Can you work these out from the model? Positions are in its coordinate system, mm. A direction names the side the tool comes from. Give positions to 0.01 mm unless a question says otherwise; leave off trailing zeros. Loops run counter-clockwise (first coordinate to the right, second up) from the corner with the lowest first, then second, coordinate; pieces in that order, holes last. Notation, with made-up numbers: (13.25, 78) - (63.25, 78) arc R18 ccw to (63.25, 85) - close; hole circle Ø11 at (43, -21). An arc over 180 degrees is marked (long way). Write item = value, one per line.
from build123d import *

# Parameters (mm, degrees)
F0_R        = 2.61
F1_DEPTH    = 15
F2_R        = 7.5
F2_R_2      = 2.61
F3_DEPTH    = 5
F4_R        = 7.5
F4_R_2      = 2.61
F5_DEPTH    = 13.5
F6_R        = 7.5
F6_R_2      = 2.61
F7_DEPTH    = 21
F8_C1_SIZE2 = 0.5
F8_C1_SIZE  = 1
F8_C2_SIZE2 = 0.5
F8_C2_SIZE  = 1
F8_C3_SIZE2 = 1
F8_C3_SIZE  = 0.5
F8_C4_SIZE2 = 1
F8_C4_SIZE  = 0.5
F8_C5_SIZE2 = 1
F8_C5_SIZE  = 0.5
F8_C6_SIZE2 = 0.5
F8_C6_SIZE  = 1
F9_SIZE     = 1


with BuildPart() as f1:
    # F0 (on Top) → F1 (new body)
    with BuildSketch(Plane.XY):
        with BuildLine():
            Line((20.7144641229, 7.4945626465), (6.3477137036, 32.3785043124))
            ThreePointArc((6.3477137036, 32.3785043124), (0, 43.8730669589), (-6.3477137036, 32.3785043124))
            Line((-6.3477137036, 32.3785043124), (-20.7144641229, 7.4945626465))
            ThreePointArc((-20.7144641229, 7.4945626465), (-27.4951905284, -3.75), (-14.3667504193, -3.5))
            Line((-14.3667504193, -3.5), (14.3667504193, -3.5))
            ThreePointArc((14.3667504193, -3.5), (27.4951905284, -3.75), (20.7144641229, 7.4945626465))
        make_face()
        with Locations((-21, 0)):
            Circle(F0_R, mode=Mode.SUBTRACT)
        with Locations((21, 0)):
            Circle(F0_R, mode=Mode.SUBTRACT)
        Polygon((12.3397459622, 5), (-12.3397459622, 5), (0, 26.3730669589), align=None, mode=Mode.SUBTRACT)
        with Locations((0, 36.3730669589)):
            Circle(F0_R, mode=Mode.SUBTRACT)
    extrude(amount=F1_DEPTH)

    # F2 (on face) → F3 (join)
    with BuildSketch(Plane.XY.offset(15)):
        with Locations((0, 36.3730669589)):
            Circle(F2_R)
        with Locations((0, 36.3730669589)):
            Circle(F2_R_2, mode=Mode.SUBTRACT)
    extrude(amount=F3_DEPTH)

    # F4 (on face) → F5 (join)
    with BuildSketch(Plane.XY.offset(15)):
        with Locations((21, 0)):
            Circle(F4_R)
        with Locations((21, 0)):
            Circle(F4_R_2, mode=Mode.SUBTRACT)
    extrude(amount=F5_DEPTH)

    # F6 (on face) → F7 (join)
    with BuildSketch(Plane.XY.offset(15)):
        with Locations((-21, 0)):
            Circle(F6_R)
        with Locations((-21, 0)):
            Circle(F6_R_2, mode=Mode.SUBTRACT)
    extrude(amount=F7_DEPTH)

    # F8: chamfer of 0.5 x 1 on 6 edges, made by hand

    # F8_c1
    f8_c1_edges = [f1.edges().sort_by_distance(p)[0] for p in [
        (-23.61, 0, 36),
    ]]
    f8_c1_side = f1.faces().sort_by_distance((-23.62, 0, 36))[0]
    chamfer(f8_c1_edges, length=F8_C1_SIZE, length2=F8_C1_SIZE2, reference=f8_c1_side)

    # F8_c2
    f8_c2_edges = [f1.edges().sort_by_distance(p)[0] for p in [
        (-23.61, 0, 0),
    ]]
    f8_c2_side = f1.faces().sort_by_distance((-23.61, 0, 0.01))[0]
    chamfer(f8_c2_edges, length=F8_C2_SIZE, length2=F8_C2_SIZE2, reference=f8_c2_side)

    # F8_c3
    f8_c3_edges = [f1.edges().sort_by_distance(p)[0] for p in [
        (18.39, 0, 0),
    ]]
    f8_c3_side = f1.faces().sort_by_distance((18.38, 0, 0))[0]
    chamfer(f8_c3_edges, length=F8_C3_SIZE, length2=F8_C3_SIZE2, reference=f8_c3_side)

    # F8_c4
    f8_c4_edges = [f1.edges().sort_by_distance(p)[0] for p in [
        (-2.61, 36.3730669589, 0),
    ]]
    f8_c4_side = f1.faces().sort_by_distance((-2.62, 36.3730669589, 0))[0]
    chamfer(f8_c4_edges, length=F8_C4_SIZE, length2=F8_C4_SIZE2, reference=f8_c4_side)

    # F8_c5
    f8_c5_edges = [f1.edges().sort_by_distance(p)[0] for p in [
        (-2.61, 36.3730669589, 20),
    ]]
    f8_c5_side = f1.faces().sort_by_distance((-2.61, 36.3730669589, 19.99))[0]
    chamfer(f8_c5_edges, length=F8_C5_SIZE, length2=F8_C5_SIZE2, reference=f8_c5_side)

    # F8_c6
    f8_c6_edges = [f1.edges().sort_by_distance(p)[0] for p in [
        (18.39, 0, 28.5),
    ]]
    f8_c6_side = f1.faces().sort_by_distance((18.39, 0, 28.49))[0]
    chamfer(f8_c6_edges, length=F8_C6_SIZE, length2=F8_C6_SIZE2, reference=f8_c6_side)

    # F9
    f9_edges = [f1.edges().sort_by_distance(p)[0] for p in [
        (6.169873, 15.686533, 0),
        (0, 5, 0),
        (-6.169873, 15.686533, 0),
        (0, -3.5, 0),
        (-13.531089, 19.936533, 0),
        (13.531089, 19.936533, 0),
    ]]
    chamfer(f9_edges, length=F9_SIZE)


solid = f1.part
Q1. Imagine slicing it at D-D, the plane z = 25. Write out the boundary of the cut face in (x, y).
Output:
outline = circle Ø15 at (-21, 0); circle Ø15 at (21, 0); hole circle Ø5.22 at (-21, 0); hole circle Ø5.22 at (21, 0)
Q2. I need wall thicknesses on L1, parallel to Y at x = 21, z = 8; L2, parallel to X at y = -2, z = 12.5; L3, parallel to Z at x = 4, y = 26.5. Which ranges of each line are inside material? Lowest first, please.
Output:
L1 = -7.5 to -2.61, 2.61 to 7.5
L2 = -28.23 to -22.68, -19.32 to 19.32, 22.68 to 28.23
L3 = 0 to 15
Q3. We'd pull the mould along Y, two halves only. Please class faces 6 (the flat face through (0, -3.5, 8)), 7 (the flat face through (-5, 19, 15)), 8 (the cylindrical face through (-23.607, 0.115, 18.008)): released by +Y, released by -Y, zero draft, split by the parting line, or undercut.
Output:
face_6 = released by -Y
face_7 = zero draft
face_8 = undercut
Q4. Imagine slicing it at A-A, the plane y = 0. Write out the boundary of the cut face in (x, z).
Output:
outline = (-28.5, 0) - (-24.11, 0) - (-23.61, 1) - (-23.61, 35.5) - (-24.61, 36) - (-28.5, 36) - close; (-18.39, 1) - (-17.89, 0) - (17.89, 0) - (18.39, 1) - (18.39, 27.5) - (17.89, 28.5) - (13.5, 28.5) - (13.5, 15) - (-13.5, 15) - (-13.5, 36) - (-17.39, 36) - (-18.39, 35.5) - close; (23.61, 1) - (24.11, 0) - (28.5, 0) - (28.5, 28.5) - (24.11, 28.5) - (23.61, 27.5) - close
Q5. Which directions (+Z, -Z, +X, -X, +Y, -Y) give clear straight access to the entire face, cutting with the end or side of a thin tool? Please do faces 1 (the flat face through (-6.5, 18.3, 0)), 2 (the flat face through (24, -2, 28.5)), 3 (the flat face through (-6.256, 15.537, 7.902)), 4 (the flat face through (-2, 33, 20)), 5 (the flat face through (6.5, 16.1, 0.51)).
Output:
face_1 = -Z, +X, -X, +Y, -Y
face_2 = +Z, +X, +Y, -Y
face_3 = +Z, -Z
face_4 = +Z, +X, -X, +Y, -Y
face_5 = -Z
Q6. Imagine slicing it at C-C, the plane x = 8.5. Write out the boundary of the cut face in (y, z).
Output:
outline = (-3.5, 1) - (-2.5, 0) - (4, 0) - (5, 1) - (5, 15) - (-3.5, 15) - close; (11.65, 1) - (13.65, 0) - (26.65, 0) - (28.65, 1) - (28.65, 15) - (11.65, 15) - close
Q7. For pin 1 (16.5 mm diameter, centred on x = -2, y = 39, fed in from +Z); pin 2 (15.5 mm diameter, centred on x = 3, z = 5, fed in from -Y); pin 3 (10 mm diameter, centred on x = 20.5, z = 14.5, fed in from +Y), each with a flat end and sliding along its axis, tell me the tip position at first contact or that it passes through.
Output:
pin_1 = 20
pin_2 = -3.5
pin_3 = 16.53
Q8. Imagine slicing it at B-B, the plane z = 16. Write out the boundary of the cut face in (x, y), then the cut area to 3 significant figures.
Output:
outline = circle Ø15 at (-21, 0); circle Ø15 at (0, 36.37); circle Ø15 at (21, 0); hole circle Ø5.22 at (-21, 0); hole circle Ø5.22 at (0, 36.37); hole circle Ø5.22 at (21, 0)
area = 466 mm2
